Can you work these out from the model? Positions are in its coordinate system, mm. A direction names the side the tool comes from. Round coordinates to 2 decimals unless told otherwise and drop trailing zeros. Order: outer loops, then holes, each group sorted by start corner. A loop starts at its lowest first (then second) coordinate and runs counter-clockwise, first axis right, second up. Notation, with made-up numbers: M 22,-14 L 81,-14 A8 ccw 81,-6 Z; hole C 5,59.25 d10. An arc over 180 degrees is marked long. One line per question, with ' | ' between items.
```python
from build123d import *

# Parameters (mm, degrees)
F0_R     = 1.5875
F1_DEPTH = 3.048


with BuildPart() as f1:
    # F0 (on Front) → F1 (new body)
    with BuildSketch(Plane.XZ):
        with BuildLine():
            Line((-9.525, 50.8), (-15.747457, 2.008289))
            ThreePointArc((-15.747457, 2.008289), (-15.851677, -0.860203), (-15.437661, -3.700573))
            Line((-15.437661, -3.700573), (-9.525, -63.5))
            ThreePointArc((-9.525, -63.5), (-6.613434, -70.354788), (0.341271, -73.018884))
            Line((0.341271, -73.018884), (44.45, -71.4375))
            ThreePointArc((44.45, -71.4375), (52.3875, -63.5), (44.45, -55.5625))
            Line((44.45, -55.5625), (18.890116, -54.646128))
            ThreePointArc((18.890116, -54.646128), (13.188544, -51.932521), (11.263342, -45.918772))
            Line((11.263342, -45.918772), (15.437661, -3.700573))
            ThreePointArc((15.437661, -3.700573), (15.765286, -1.863163), (15.875, 0))
            Line((15.875, 0), (15.386538, 3.907692))
            Line((15.386538, 3.907692), (9.525, 50.8))
            ThreePointArc((9.525, 50.8), (0, 60.325), (-9.525, 50.8))
        make_face()
        with Locations((0, -63.5)):
            Circle(F0_R, mode=Mode.SUBTRACT)
        with Locations((44.45, -63.5)):
            Circle(F0_R, mode=Mode.SUBTRACT)
        with Locations((-4.372607, 37.063282)):
            Circle(F0_R, mode=Mode.SUBTRACT)
        with Locations((0, 50.8)):
            Circle(F0_R, mode=Mode.SUBTRACT)
    extrude(amount=F1_DEPTH)


solid = f1.part
```
(1) If we section it at B-B on x = 28: Please give me the cut outline in (y, z).
Final values:
outline: M -3.05,-72.03 L 0,-72.03 L 0,-54.97 L -3.05,-54.97 Z
(2) Please list where these lines run through material, in increasing order: probe 1 along Z at (x, y) = (0, -0.6) (1 decimal); probe 2 along Z at (x, y) = (44.45, -1.45); probe 3 along Z at (x, y) = (45, -0.3). Write a range as [from, to].
Final values:
probe 1: [-73, -65.1], [-61.9, 49.2], [52.4, 60.3] | probe 2: [-71.44, -65.09], [-61.91, -55.56] | probe 3: [-71.42, -64.99], [-62.01, -55.58]
(3) Will this pin go through, and if not, where does the flat tip stop? pin 1 Ø3 at (x, z) = (0, 50.8) entering from -Y.
Final values:
pin 1: through
(4) If we section it at C-C on z = 47.5: Please give me the cut outline in (x, y).
Final values:
outline: M -9.95,-3.05 L 9.94,-3.05 L 9.94,0 L -9.95,0 Z
(5) On a 3-axis mill with a long thin cutter (end or side, diameter ignored), from which of +Z, -Z, +X, -X, +Y, -Y can I reach the whole of each face in a straight line? I mean faces 1 (the cylindrical face through (13.25, -1.5, -52)), 2 (the cylindrical face through (-3.519, -1.503, 38.402)). Say none if no direction works.
Final values:
face 1: +X, +Y, -Y | face 2: +Y, -Y
(6) If we section it at A-A on x = -4: Please give me the cut outline in (y, z).
Final values:
outline: M -3.05,-72.14 L 0,-72.14 L 0,35.52 L -3.05,35.52 Z; M -3.05,38.61 L 0,38.61 L 0,59.44 L -3.05,59.44 Z
(7) Thinking about a two-plate mould opening in X: for faces 3 (the flat face through (-12.523, -1.503, -33.182)), 4 (the cylindrical face through (44.243, -1.503, -61.926)), 5 (the cylindrical face through (15.762, -1.503, -1.889)), which applies, released by +X, released by -X, zero draft, split by the parting line, or undercut?
Final values:
face 3: released by -X | face 4: undercut | face 5: released by +X
